```python
from build123d import *

# Parameters (mm, degrees)
F1_DEPTH    = 22.86
F3_DEPTH    = 22.861
F5_DEPTH    = 21.1407149532
F6_R        = 0.9322227143
F7_DEPTH    = 21.1407149532
F8_R        = 1.27
F9_T4_DEPTH = 16.1477728221


# Not quite as in the source:
# - a fillet or chamfer that OpenCascade refuses, or shapes differently, is made with other operations: its cross-section is extruded or revolved along the edge and cut away or added
# - a feature names something its author has since deleted; it is built from what else it names


with BuildPart() as f1:
    # F0 (on Right) → F1 (new body)
    with BuildSketch(Plane.YZ):
        Polygon((0, 5.6908354163), (-12.0390886441, 11.6551341489), (-5.6838279371, 0), (-8.9875673875, -9.0952031314), (0, -5.6768290866), (12.0390886441, -11.6551341489), (5.6978515349, 0), (8.9875673875, 9.0952031314), align=None)
    extrude(amount=F1_DEPTH)

    # F2 (on face) → F3 (cut, through all)
    with BuildSketch(Plane.YZ.offset(22.86)):
        Polygon((0.2947798819, -4.2920547475), (4.8379492509, -6.9700027277), (4.4653764926, -4.1452315636), align=None)
        Polygon((-0.460864554, -3.1500807424), (4.8379492509, -3.1500807424), (4.2156420195, -0.4934913878), align=None)
        Polygon((-6.4040375873, -6.2635522336), (-1.3339594007, -5.0133955665), (-2.1420896955, -3.1500807424), (-3.6510264616, -2.3839071877), align=None)
        Polygon((-3.6510264616, 0.7806772021), (-1.3339594007, 1.3762915041), (-1.4712439905, 4.1567722153), (-3.6510264616, 6.1231630373), align=None)
        Polygon((-8.9875673875, 8.8637409893), (-4.6268783625, 0.7806772021), (-4.6268783625, 5.8275670744), (-4.6572963607, 6.6916077305), align=None)
        Polygon((0.9543706066, -0.4934913878), (4.4653764926, 0.9595727897), (5.9346228684, 5.0216543911), align=None)
        Polygon((0, 1.3762915041), (5.1912929219, 6.1231630373), (0, 4.1567722153), align=None)
        Polygon((-0.1954076109, -0.4954853684), (-4.0261200629, 0), (-1.1355356546, -2.0616382826), align=None)
        Polygon((8.1868149158, -8.1874002878), (6.6878763027, -4.839763511), (6.3406112604, -7.2706225328), align=None)
    extrude(amount=-F3_DEPTH, mode=Mode.SUBTRACT)

    # F4 (on face) → F5 (cut, through all)
    with BuildSketch(Plane(origin=(0, -4.381188718, -2.3889554726), x_dir=(1, 0, 0), z_dir=(0, -0.8779615957, -0.4787310691))):
        Polygon((20.7448676229, 13.0785638466), (14.3051566556, 13.0785638466), (19.5283554494, 5.3454530425), align=None)
    extrude(amount=-F5_DEPTH, mode=Mode.SUBTRACT)

    # F6 (on face) → F7 (cut, through all)
    with BuildSketch(Plane(origin=(0, -4.381188718, -2.3889554726), x_dir=(1, 0, 0), z_dir=(0, -0.8779615957, -0.4787310691))):
        with Locations((21.6227080673, 14.5550044253)):
            Circle(F6_R)
    extrude(amount=-F7_DEPTH, mode=Mode.SUBTRACT)

    # F8
    f8_edges = [f1.edges().sort_by_distance(p)[0] for p in [
        (0, -8.861458, 5.827567),
    ]]
    fillet(f8_edges, radius=F8_R)

    # F9: chamfer of 1.27 on 1 edges, made by hand


with BuildPart() as f9_tool2:
    # F9_s3 → F9_t4 (new body)
    with BuildSketch(Plane(origin=(0, -13.9265349188, -5.2968844013), x_dir=(1, 0, 0), z_dir=(0, 0.9346765421, 0.355499313))):
        Polygon((0, 4.035998981), (1.27, 5.305998981), (0, 5.305998981), align=None)
    extrude(amount=F9_T4_DEPTH)

    split(bisect_by=Plane(origin=(0, -2.2613507756, -4.553899836), x_dir=(1, 0, 0), z_dir=(0, -0.4447575076, -0.8956510255)), keep=Keep.TOP)


with BuildPart() as f1_1:
    add(f1.part)

    # F9_t1: cut F9_tool2
    add(f9_tool2.part, mode=Mode.SUBTRACT)


solid = f1_1.part
```
The model under review builds one solid part; all positions refer to its coordinate system, in mm. A direction names the side the tool comes from. Give positions to 0.01 mm unless a question says otherwise; leave off trailing zeros.
(1) For P1, Ø2, axis at x = 2.5, y = -4.5, coming from the -Z side; P2, Ø0.8, axis at x = 9, z = 3.5, coming from the +Y side; P3, Ø3, axis at y = 6, z = -9, coming from the +X side; P4, Ø6, axis at x = 2.5, z = -8.5, coming from the -Y side, all flat-tipped, find the tip position at first contact; note any pin that passes through.
(2) The part is to be moulded in two halves that separate along Y. For faces 5 (the flat face through (11.27, 7.32, 4.48)), 6 (the flat face through (11.59, -5.01, -4.3)), 7 (the flat face through (11.27, -7.45, -4.86)), say which applies: released by +Y, released by -Y, zero draft, split by the parting line, or undercut.
(3) Consider section A-A, the plane x = 16.5. Give the number of separate pieces and of enclosed holes in the cut face, and give its area (3 significant figures).
(4) Tool access review of faces 1 (the flat face through (11.59, 2.53, -5.61)), 2 (the flat face through (11.27, 8.913, -5.909)), 3 (the flat face through (11.27, 4.56, 7.42)), 4 (the cylindrical face through (21.42, -10.31, 9.92)): name each direction out of +Z, -Z, +X, -X, +Y, -Y from which nothing blocks a thin tool from reaching the whole face with its end or side.
(5) To check wall thickness, follow L1, parallel to Z at x = 3.5, y = -2.5; L2, parallel to Y at x = 5.5, z = 3; L3, parallel to Z at x = 2, y = 2.25. State the ranges of each line that lie inside material, in increasing order.
Returned:
1. P1: stops at z = -7.77
1. P2: stops at y = 7.11
1. P3: stops at x = 22.86
1. P4: stops at y = -8.99
2. face 5: released by +Y
2. face 6: undercut
2. face 7: released by -Y
3. separate pieces: 2
3. enclosed holes: 8
3. area: 166 mm2
4. face 1: +X, -X
4. face 2: +X, -X, +Y
4. face 3: +Z, +X, -X
4. face 4: none
5. L1: z = -6.63 to -5.3, -2.97 to -1.09, -0.2 to 1.08, 5.08 to 6.93
5. L2: y = -7.32 to -5.82, -4.63 to -3.65, -1.41 to 0, 1.78 to 4.11, 5.2 to 6.78
5. L3: z = -6.79 to -5.44, -4.22 to -3.15, -1.61 to 0.04, 0.94 to 3.43, 5.01 to 6.54
